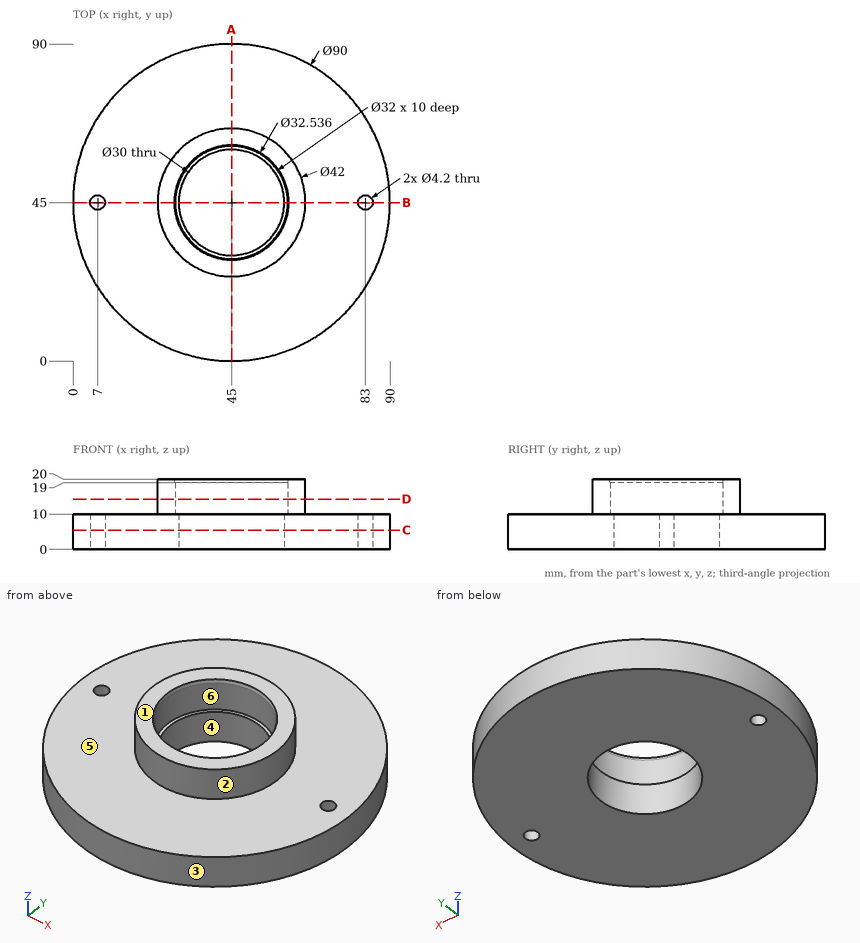
Check sheet for the drawn part. Datum: minimum x, y, z corner. Units: mm. A direction names the side the tool comes from. Round coordinates to 2 decimals unless told otherwise and drop trailing zeros. Loops run counter-clockwise (first coordinate to the right, second up) from the corner with the lowest first, then second, coordinate; pieces in that order, holes last. Notation, with made-up numbers: (52, 10) - (72, 10) arc R33 cw to (72, 44) - close; hole circle Ø7 at (-31.5, 87.5). An arc over 180 degrees is marked (long way). Write item = value, one per line. Start each with the question number.
1. Section check C-C on z = 5.5. Enter the section's corners in (x, y).
2. Section check B-B on y = 45. Enter the section's corners in (x, z).
3. Section check A-A on x = 45. Enter the section's corners in (y, z), then the cut area to 3 significant figures.
4. Thickness scan on line 1 (Y direction, x = 45, z = 5.75); line 2 (X direction, y = 45.5, z = 2); line 3 (Z direction, x = 42, y = 10). Record the ranges inside material, lowest first.
5. Set-up check for the marked faces 1 and 2: record each of +Z, -Z, +X, -X, +Y, -Y from which the full face is reachable in a straight line by a thin tool's end or side.
6. Mould release check, pull along Y, two halves, no side actions. Record for the marked faces 3, 4, 5 and 6: released by +Y, released by -Y, zero draft, split by the parting line, or undercut.
7. Depth check by flat-ended pin: pin 1 (5 mm diameter, centred on x = 25, z = 3.5, fed in from +Y); pin 2 (1 mm diameter, centred on y = 34.5, z = 16.5, fed in from -X); pin 3 (3 mm diameter, centred on y = 69, z = 5.5, fed in from -X); pin 4 (12 mm diameter, centred on x = 60, y = 28.5, fed in from +Z). Enter the tip coordinate at first touch or a pass-through.
8. Section check D-D on z = 14.25. Enter the section's corners in (x, y), then the cut area to 3 significant figures.
Working result:
q1.outline = circle Ø90 at (45, 45); hole circle Ø4.2 at (7, 45); hole circle Ø30 at (45, 45); hole circle Ø4.2 at (83, 45)
q2.outline = (0, 0) - (4.9, 0) - (4.9, 10) - (0, 10) - close; (9.1, 0) - (30, 0) - (30, 10) - (29, 10) - (29, 19) - (28.73, 20) - (24, 20) - (24, 10) - (9.1, 10) - close; (60, 0) - (80.9, 0) - (80.9, 10) - (66, 10) - (66, 20) - (61.27, 20) - (61, 19) - (61, 10) - (60, 10) - close; (85.1, 0) - (90, 0) - (90, 10) - (85.1, 10) - close
q3.outline = (0, 0) - (30, 0) - (30, 10) - (29, 10) - (29, 19) - (28.73, 20) - (24, 20) - (24, 10) - (0, 10) - close; (60, 0) - (90, 0) - (90, 10) - (66, 10) - (66, 20) - (61.27, 20) - (61, 19) - (61, 10) - (60, 10) - close
q3.area = 700 mm^2
q4.line_1 = 0 to 30, 60 to 90
q4.line_2 = 0 to 4.96, 9.04 to 30.01, 59.99 to 80.96, 85.04 to 90
q4.line_3 = 0 to 10
q5.face_1 = +Z, +X, -X, +Y, -Y
q5.face_2 = +Z
q6.face_3 = split by the parting line
q6.face_4 = undercut
q6.face_5 = zero draft
q6.face_6 = undercut
q7.pin_1 = 86.46
q7.pin_2 = 26.53
q7.pin_3 = 6.03
q7.pin_4 = 20
q8.outline = circle Ø42 at (45, 45); hole circle Ø32 at (45, 45)
q8.area = 581 mm^2
